The listing builds one solid part. Answer for the finished solid, in the listing's coordinates (mm). Round coordinates to 2 decimals unless told otherwise and drop trailing zeros. Write each loop counter-clockwise with the first axis right and the second up, starting at its lowest first coordinate (ties: lowest second). Pieces come first, ordered by that corner, then holes.
from build123d import *

# Parameters (mm, degrees)
F0_W     = 3
F0_H     = 2
F0_W_2   = 4
F0_H_2   = 2.991964
F1_DEPTH = 5.5


with BuildPart() as f1:
    # F0 (on Top) → F1 (new body)
    with BuildSketch(Plane.XY):
        Polygon((-36.408239, -50.416655), (-40.408239, -50.416655), (-40.408239, -73.416655), (-36.408239, -73.416655), (-36.408239, -70.416655), (-36.408239, -52.416655), align=None)
        with Locations((-34.908239, -51.416655)):
            Rectangle(F0_W, F0_H)
        with Locations((-38.408239, -74.416655)):
            Rectangle(F0_W_2, F0_H)
        Polygon((-36.408239, -70.416655), (-36.408239, -73.416655), (77.031761, -73.416655), (77.031761, -73.408619), (77.031761, -70.416655), (73.57222, -70.416655), align=None)
        Polygon((77.031761, -73.408619), (77.031761, -73.416655), (77.031761, -75.408619), (81.031761, -75.453453), (81.031761, -73.408619), align=None)
        Polygon((73.57222, -50.416655), (73.57222, -70.416655), (77.031761, -70.416655), (77.031761, -48.309352), (73.952891, -37.865963), (73.952891, -35.947701), (65.952891, -35.947701), (65.994848, -37.94726), (69.896053, -37.94726), align=None)
        with Locations((79.031761, -71.912637)):
            Rectangle(F0_W_2, F0_H_2)
        Polygon((81.031761, -70.416655), (81.031761, -73.408619), (81.031761, -75.453453), (82.42857, -80.254382), (80.92857, -80.254382), (81.617752, -82.131888), (84.117752, -82.131888), align=None)
    extrude(amount=F1_DEPTH)


solid = f1.part
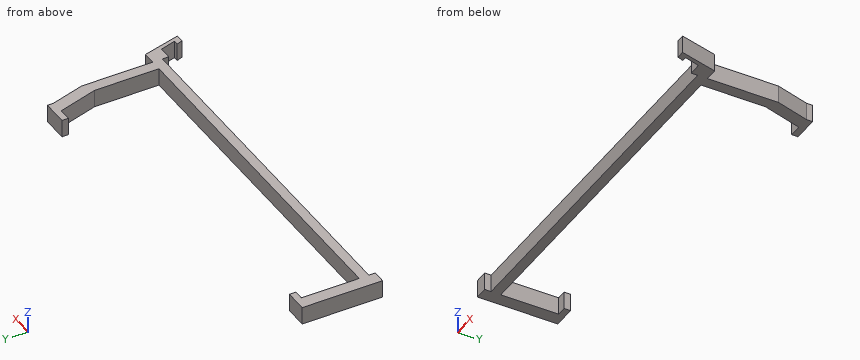
1. Straight lines are drawn through the part: line 1 along Y through (x, z) = (21.5, 5); line 2 along X through (y, z) = (-53, 3.35); line 3 along X through (y, z) = (-73.5, 0.6). For each, find the intervals that lie inside material, in ascending order.
Geometry says:
line 1: y = -73.42 to -70.42
line 2: x = -40.41 to -36.41, 73.57 to 77.03
line 3: x = -40.41 to -36.41, 77.03 to 81.84
2. Given pin 1 (1.5 mm diameter, centred on y = -36.5, z = 4, fed in from +X); pin 2 (12 mm diameter, centred on x = -3, y = -70, fed in from -Z); pin 3 (3 mm diameter, centred on x = 68, z = 3.5, fed in from -Y); pin 4 (1.6 mm diameter, centred on y = -74.5, z = 3, fed in from +X), each flat-ended and moving along its own axis, determine where each tip first touches the part or whether it passes through.
Geometry says:
pin 1: stops at x = 73.95
pin 2: stops at z = 0
pin 3: stops at y = -73.42
pin 4: stops at x = 82.32
3. Section B-B on z = 3.3 is taken. Determine the outline of the cut face in (x, y), plus the area to 3 significant figures.
Geometry says:
outline: (-40.41, -75.42) - (-36.41, -75.42) - (-36.41, -73.42) - (77.03, -73.42) - (77.03, -75.41) - (81.03, -75.45) - (82.43, -80.25) - (80.93, -80.25) - (81.62, -82.13) - (84.12, -82.13) - (81.03, -70.42) - (77.03, -70.42) - (77.03, -48.31) - (73.95, -37.87) - (73.95, -35.95) - (65.95, -35.95) - (65.99, -37.95) - (69.9, -37.95) - (73.57, -50.42) - (73.57, -70.42) - (-36.41, -70.42) - (-36.41, -52.42) - (-33.41, -52.42) - (-33.41, -50.42) - (-40.41, -50.42) - close
area: 616 mm2
4. Section C-C on x = -25.5 is taken. Determine the outline of the cut face in (y, z), plus the area to 3 significant figures.
Geometry says:
outline: (-73.42, 0) - (-70.42, 0) - (-70.42, 5.5) - (-73.42, 5.5) - close
area: 16.5 mm2
5. Section A-A on y = -68 is taken. Determine the outline of the cut face in (x, z).
Geometry says:
outline: (-40.41, 0) - (-36.41, 0) - (-36.41, 5.5) - (-40.41, 5.5) - close; (73.57, 0) - (77.03, 0) - (77.03, 5.5) - (73.57, 5.5) - close
